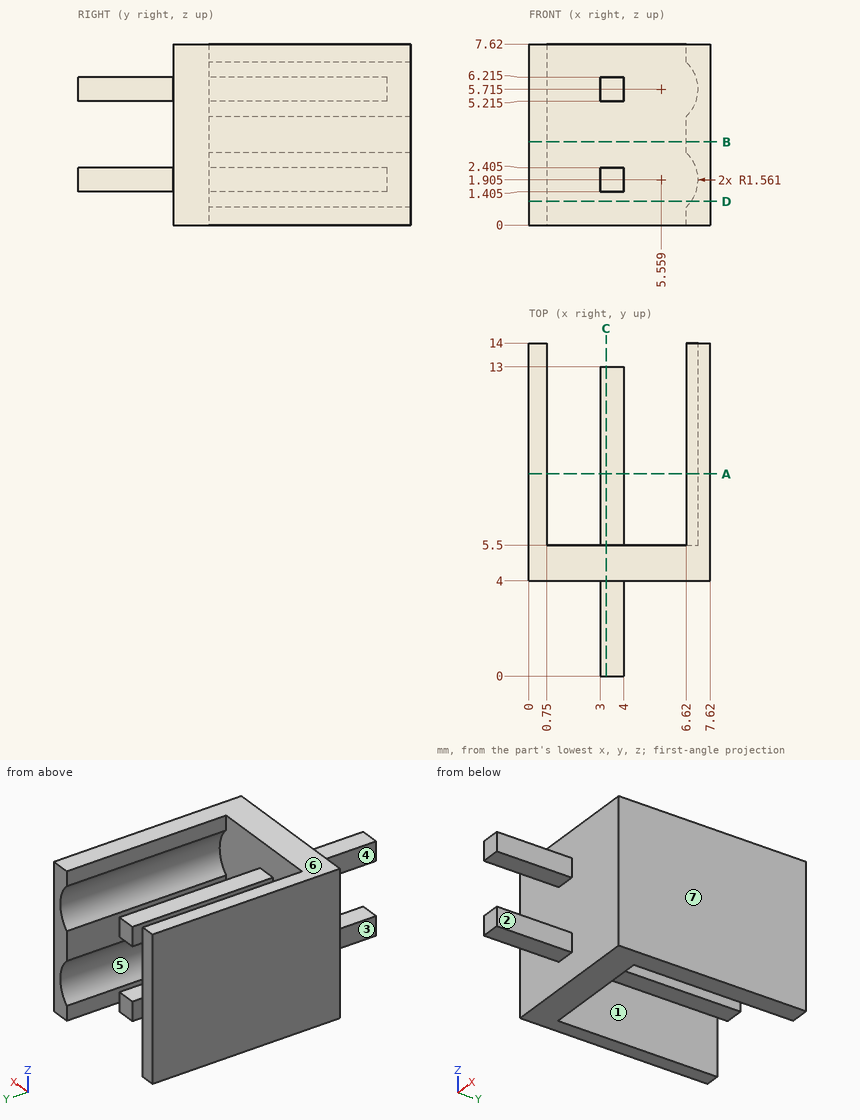
Input: dimensioned drawing with shaded views. Units: mm. Origin: part minimum x, y, z. A direction names the side the tool comes from. Coordinates: 2 decimals unless noted, no trailing zeros. Loops run counter-clockwise (first coordinate to the right, second up) from the corner with the lowest first, then second, coordinate; pieces in that order, holes last. Notation, with made-up numbers: M 3,46.5 L 9,46.5 A12 ccw 9,53.5 Z; hole C 75,9.25 d7. An arc over 180 degrees is marked long. One line per item, written item: value.
(1) Section C-C (x = 3.25). Output: boundary loops of the cut face in (y, z) (1 decimal).
Filled in:
outline: M 0,1.4 L 4,1.4 L 4,0 L 5.5,0 L 5.5,1.4 L 13,1.4 L 13,2.4 L 5.5,2.4 L 5.5,5.2 L 13,5.2 L 13,6.2 L 5.5,6.2 L 5.5,7.6 L 4,7.6 L 4,6.2 L 0,6.2 L 0,5.2 L 4,5.2 L 4,2.4 L 0,2.4 Z
(2) Section A-A (y = 8.5). Give the number of separate pieces and of enclosed holes in the cut face.
Filled in:
separate pieces: 4
enclosed holes: 0
(3) Section D-D (z = 1). Output: boundary loops of the cut face in (x, y).
Filled in:
outline: M 0,4 L 7.62,4 L 7.62,14 L 6.83,14 L 6.83,5.5 L 0.75,5.5 L 0.75,14 L 0,14 Z
(4) Pin query (flat end, axial travel): pin 1 (2 mm diameter, centred on x = 6, z = 4.5, fed in from +Y); pin 2 (1.1 mm diameter, centred on x = 3.5, z = 5.5, fed in from +Y); pin 3 (0.8 mm diameter, centred on x = 3.5, y = 1.5, fed in from -Z) (3 decimals); pin 4 (1.1 mm diameter, centred on x = 3.5, y = 10.5, fed in from +Z) (3 decimals). Return the tip coordinate at first contact, or that it passes through.
Filled in:
pin 1: y = 14
pin 2: y = 13
pin 3: z = 1.405
pin 4: z = 6.215
(5) Line query: line 1 along X through (y, z) = (12, 3.5); line 2 along Z through (x, y) = (3.25, 8.25) (1 decimal); line 3 along Y through (x, z) = (2.75, 6). Output: solid intervals per line, ascending. Write a range as from..to.
Filled in:
line 1: 0..0.75, 6.62..7.62
line 2: 1.4..2.4, 5.2..6.2
line 3: 4..5.5
(6) Section B-B (z = 3.5). Output: boundary loops of the cut face in (x, y).
Filled in:
outline: M 0,4 L 7.62,4 L 7.62,14 L 6.62,14 L 6.62,5.5 L 0.75,5.5 L 0.75,14 L 0,14 Z
(7) Pull-direction query (X, two-part tool) for the marked faces 4, 5, 6 and 7; classes: +X half, -X half, draft (parallel to the pull), parting line (faces both ways), or undercut.
Filled in:
face 4: -X half
face 5: undercut
face 6: draft
face 7: +X half
(8) Reachability of the marked faces 1, 2 and 3 from +Z, -Z, +X, -X, +Y, -Y: full face, straight path, thin tool, end or side. Return the list, or none.
Filled in:
face 1: +Z, -Z, +Y
face 2: +Z, -Z, +X, -Y
face 3: +Z, -Z, -X, -Y
